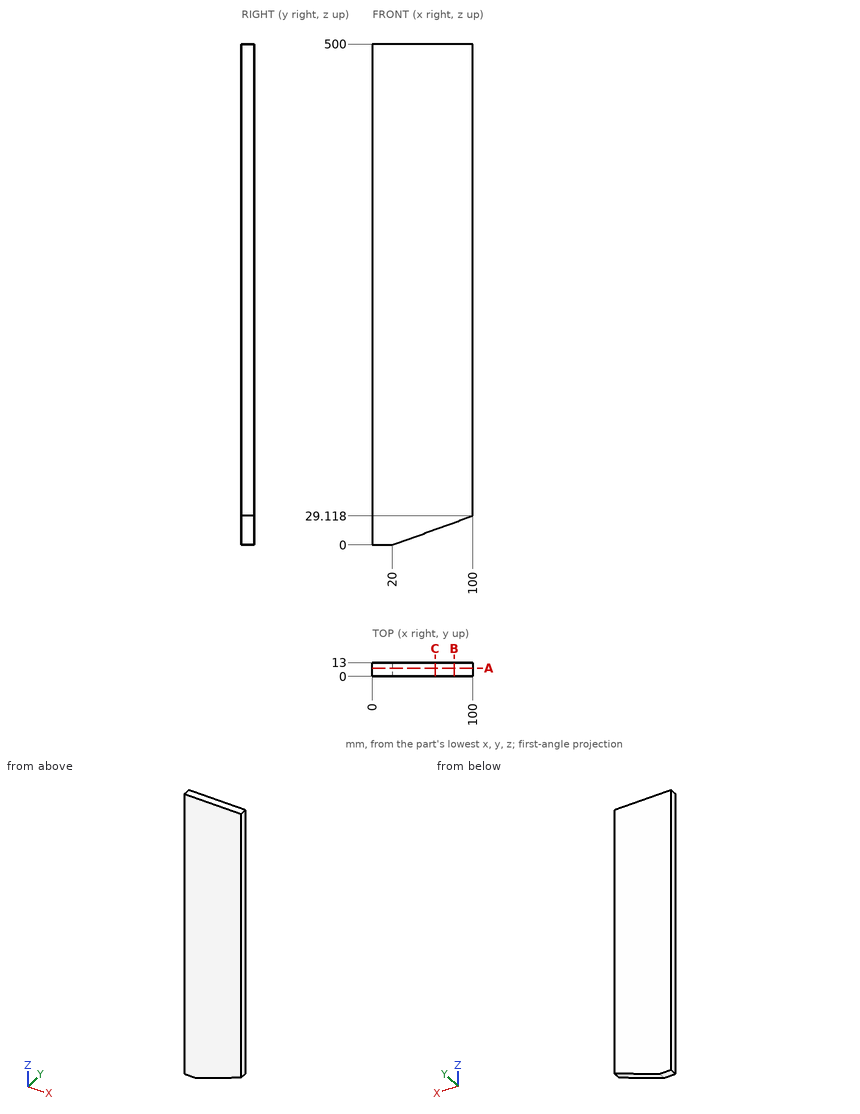
Source: three-view drawing plus pictorial views. Frame: mm from the lowest corner of the part. Round coordinates to 2 decimals unless told otherwise and drop trailing zeros. Order: outer loops, then holes, each group sorted by start corner. A loop starts at its lowest first (then second) coordinate and runs counter-clockwise, first axis right, second up. Notation, with made-up numbers: (30.25, -30) -> (75.25, -30) arc R11 ccw to (75.25, -20) -> close; hole circle Ø4 at (21, 56.5). An arc over 180 degrees is marked (long way). Use CSV: the item, a comma, the result in double quotes. Start each with the question number.
1) Section C-C (x = 62.5). Return the cut outline in (y, z).
2) First-contact query: pin 1 Ø3 at (x, y) = (63.5, 5.5) entering from -Z. Flat tip, straight axial feed; report the tip coordinate or a pass-through.
3) Section B-B (x = 81.5). Return the cut outline in (y, z).
4) Section A-A (y = 7.75). Return the cut outline in (x, z), and give its area (3 significant figures).
5) Material intervals for line 1 along Z through (x, y) = (88, 7); line 2 along Z through (x, y) = (40, 6.5), sorted ascending. Write a range as from..to.
Returned:
1,outline,"(0, 15.47) -> (13, 15.47) -> (13, 500) -> (0, 500) -> close"
2,pin 1,"stops at z = 15.29"
3,outline,"(0, 22.38) -> (13, 22.38) -> (13, 500) -> (0, 500) -> close"
4,outline,"(0, 0) -> (20, 0) -> (100, 29.12) -> (100, 500) -> (0, 500) -> close"
4,area,"48,800 mm²"
5,line 1,"z = 24.75..500"
5,line 2,"z = 7.28..500"
